```python
from build123d import *

# Parameters (mm, degrees)
SKETCH1_W                                            = 70
SKETCH1_H                                            = 100
BOSS_EXTRUDE1_DEPTH                                  = 10
SKETCH2_R                                            = 2.5
CUT_EXTRUDE1_DEPTH                                   = 11
SKETCH3_R                                            = 1.5
CUT_EXTRUDE2_DEPTH                                   = 11
SKETCH5_R                                            = 2
CUT_EXTRUDE4_DEPTH                                   = 11
CSK_FOR_M4_SOCKET_COUNTERSUNK_HEAD_SCREW_D           = 4.5
CSK_FOR_M4_SOCKET_COUNTERSUNK_HEAD_SCREW_CSINK_D     = 9.18
CSK_FOR_M4_SOCKET_COUNTERSUNK_HEAD_SCREW_CSINK_ANGLE = 90
CSK_FOR_M5_SOCKET_COUNTERSUNK_HEAD_SCREW_D           = 5.5
CSK_FOR_M5_SOCKET_COUNTERSUNK_HEAD_SCREW_CSINK_D     = 11.47
CSK_FOR_M5_SOCKET_COUNTERSUNK_HEAD_SCREW_CSINK_ANGLE = 90


with BuildPart() as part:
    # Sketch1 → Boss-Extrude1 (new body)
    with BuildSketch(Plane.XY):
        Rectangle(SKETCH1_W, SKETCH1_H)
    extrude(amount=BOSS_EXTRUDE1_DEPTH)

    # Sketch2 → Cut-Extrude1 (cut, through all)
    with BuildSketch(Plane(origin=(0, 0, 0), x_dir=(-1, 0, 0), z_dir=(0, 0, -1))):
        with Locations((-25, 45)):
            Circle(SKETCH2_R)
        with Locations((25, 45)):
            Circle(SKETCH2_R)
        with Locations((-25, -45)):
            Circle(SKETCH2_R)
        with Locations((25, -45)):
            Circle(SKETCH2_R)
    extrude(amount=-CUT_EXTRUDE1_DEPTH, mode=Mode.SUBTRACT)

    # Sketch3 → Cut-Extrude2 (cut, through all)
    with BuildSketch(Plane(origin=(0, 0, 0), x_dir=(-1, 0, 0), z_dir=(0, 0, -1))):
        with Locations((9, 21)):
            Circle(SKETCH3_R)
        with Locations((9, 45)):
            Circle(SKETCH3_R)
        with Locations((-9, 21)):
            Circle(SKETCH3_R)
        with Locations((-9, 45)):
            Circle(SKETCH3_R)
        with Locations((9, -45)):
            Circle(SKETCH3_R)
        with Locations((9, -21)):
            Circle(SKETCH3_R)
        with Locations((-9, -45)):
            Circle(SKETCH3_R)
        with Locations((-9, -21)):
            Circle(SKETCH3_R)
    extrude(amount=-CUT_EXTRUDE2_DEPTH, mode=Mode.SUBTRACT)

    # Sketch5 → Cut-Extrude4 (cut, through all)
    with BuildSketch(Plane.XY.offset(10)):
        with Locations((0, -11)):
            Circle(SKETCH5_R)
        with Locations((0, 11)):
            Circle(SKETCH5_R)
    extrude(amount=-CUT_EXTRUDE4_DEPTH, mode=Mode.SUBTRACT)

    # CSK for M4 socket countersunk head screw1 (through all)
    with Locations(Plane.XY.offset(10)):
        with Locations((-9, 45), (9, 45), (9, 21), (-9, 21), (0, 11), (0, -11), (9, -21), (-9, -21), (-9, -45), (9, -45)):
            CounterSinkHole(CSK_FOR_M4_SOCKET_COUNTERSUNK_HEAD_SCREW_D / 2, CSK_FOR_M4_SOCKET_COUNTERSUNK_HEAD_SCREW_CSINK_D / 2, counter_sink_angle=CSK_FOR_M4_SOCKET_COUNTERSUNK_HEAD_SCREW_CSINK_ANGLE)

    # CSK for M5 socket countersunk head screw2 (through all)
    with Locations(Plane(origin=(0, 0, 0), x_dir=(-1, 0, 0), z_dir=(0, 0, -1))):
        with Locations((-25, 45), (25, 45), (25, -45), (-25, -45)):
            CounterSinkHole(CSK_FOR_M5_SOCKET_COUNTERSUNK_HEAD_SCREW_D / 2, CSK_FOR_M5_SOCKET_COUNTERSUNK_HEAD_SCREW_CSINK_D / 2, counter_sink_angle=CSK_FOR_M5_SOCKET_COUNTERSUNK_HEAD_SCREW_CSINK_ANGLE)


solid = part.part
```
Model file for the job. Use its own axes, mm. Give positions to 0.01 mm unless a question says otherwise; leave off trailing zeros. Order: outer loops, then holes, each group sorted by start corner. A loop starts at its lowest first (then second) coordinate and runs counter-clockwise, first axis right, second up.
1) Pin check, flat tips, straight feed: pin 1 (6 mm diameter, centred on x = 0, y = 11, fed in from +Z); pin 2 (7 mm diameter, centred on x = -25, y = -45, fed in from -Z) (3 decimals). Stop position of each tip, or through.
2) Saw through at D-D, the plane z = 1. Count the separate pieces of the cut face and the enclosed holes in it, then the cut area to 3 significant figures.
3) Saw through at C-C, the plane x = 25. Write the cut outline in (y, z) (3 decimals), then the cut area to 3 significant figures.
4) Mould opens along X. For faces 1 (the flat face through (0, -50, 5)), 2 (the cylindrical face through (-8.71, 47.23, 3.78)) say: +X half, -X half, draft (parallel to the pull), parting line (faces both ways), or undercut.
5) Wall check: probe 1 along X at (y, z) = (-45, 4.25); probe 2 along Y at (x, z) = (9, 2.75); probe 3 along X at (y, z) = (21, 4). Give the ranges that are in metal, low to high.
6) Saw through at A-A, the plane y = 21. Write the cut outline in (x, z), then the cut area to 3 significant figures.
7) Saw through at B-B, the plane x = -9. Write the cut outline in (y, z), then the cut area to 3 significant figures.
Computed:
1. pin 1: stops at z = 8.41
1. pin 2: stops at z = 2.235
2. separate pieces: 1
2. enclosed holes: 14
2. area: 6,560 mm2
3. outline: (-50, 0.735) - (-47.75, 2.985) - (-47.75, 10) - (-50, 10) - close; (-42.25, 2.985) - (-39.265, 0) - (39.265, 0) - (42.25, 2.985) - (42.25, 10) - (-42.25, 10) - close; (47.75, 2.985) - (50, 0.735) - (50, 10) - (47.75, 10) - close
3. area: 873 mm2
4. face 1: draft
4. face 2: undercut
5. probe 1: x = -35 to -27.75, -22.25 to -11.25, -6.75 to 6.75, 11.25 to 22.25, 27.75 to 35
5. probe 2: y = -50 to -47.25, -42.75 to -23.25, -18.75 to 18.75, 23.25 to 42.75, 47.25 to 50
5. probe 3: x = -35 to -11.25, -6.75 to 6.75, 11.25 to 35
6. outline: (-35, 0) - (-11.25, 0) - (-11.25, 7.66) - (-13.59, 10) - (-35, 10) - close; (-6.75, 0) - (6.75, 0) - (6.75, 7.66) - (4.41, 10) - (-4.41, 10) - (-6.75, 7.66) - close; (11.25, 0) - (35, 0) - (35, 10) - (13.59, 10) - (11.25, 7.66) - close
6. area: 599 mm2
7. outline: (-50, 0) - (-47.25, 0) - (-47.25, 7.66) - (-49.59, 10) - (-50, 10) - close; (-42.75, 0) - (-23.25, 0) - (-23.25, 7.66) - (-25.59, 10) - (-40.41, 10) - (-42.75, 7.66) - close; (-18.75, 0) - (18.75, 0) - (18.75, 7.66) - (16.41, 10) - (-16.41, 10) - (-18.75, 7.66) - close; (23.25, 0) - (42.75, 0) - (42.75, 7.66) - (40.41, 10) - (25.59, 10) - (23.25, 7.66) - close; (47.25, 0) - (50, 0) - (50, 10) - (49.59, 10) - (47.25, 7.66) - close
7. area: 798 mm2
